from build123d import *

# Parameters (mm, degrees)
PAD002_DEPTH    = 2.5
SKETCH009_W     = 48
SKETCH009_H     = 10.5
PAD003_DEPTH    = 0.4
SKETCH008_R     = 1.4
POCKET005_DEPTH = 5
POCKET012_DEPTH = 5
PAD008_DEPTH    = 0.4


with BuildPart() as part:
    # Sketch007 (on XZ_Plane001 of Origin002) → Pad002 (new body)
    with BuildSketch(Plane.XZ):
        Polygon((50.5, 0), (50.5, 40), (27.253439, 40), (2.5, 10.5), (2.5, 0), align=None)
    extrude(amount=PAD002_DEPTH)

    # Sketch009 (on Face7 of Pad002) → Pad003 (join)
    with BuildSketch(Plane.XZ.offset(2.5)):
        with Locations((26.5, 5.25)):
            Rectangle(SKETCH009_W, SKETCH009_H)
    extrude(amount=PAD003_DEPTH)

    # Sketch008 (on Face6 of Pad002) → Pocket005 (cut)
    with BuildSketch(Plane(origin=(0, 0, 0), x_dir=(-1, 0, 0), z_dir=(0, 1, 0))):
        with Locations((-45, 4)):
            Circle(SKETCH008_R)
        with Locations((-15, 4)):
            Circle(SKETCH008_R)
    extrude(amount=-POCKET005_DEPTH, mode=Mode.SUBTRACT)

    # Sketch021 (on XZ_Plane001 of Origin002) → Pocket012 (cut)
    with BuildSketch(Plane.XZ):
        Polygon((27.253439, 40), (2.5, 10.5), (2.5, 0), (2.8, 0), (2.8, 10.5), (27.553439, 40), align=None)
    extrude(amount=POCKET012_DEPTH, mode=Mode.SUBTRACT)

    # Sketch022 (on Face4 of Pocket012) → Pad008 (join)
    with BuildSketch(Plane.XZ.offset(2.5)):
        Polygon((14.5, 10.5), (50.5, 10.5), (50.5, 14), align=None)
    extrude(amount=PAD008_DEPTH)


solid = part.part
The listing builds one solid part. Answer for the finished solid, in the listing's coordinates (mm). Round coordinates to 2 decimals unless told otherwise and drop trailing zeros. Order: outer loops, then holes, each group sorted by start corner. A loop starts at its lowest first (then second) coordinate and runs counter-clockwise, first axis right, second up. Notation, with made-up numbers: (-19, -31.5) - (5, -31.5) arc R26 cw to (5, 1.5) - close; hole circle Ø8 at (1, 2.5). An arc over 180 degrees is marked (long way). Write item = value, one per line. Start each with the question number.
1) Section A-A, the plane z = 4 is taken. Write down the section's boundary in (x, y).
2) Section C-C, the plane x = 15 is taken. Write down the section's boundary in (y, z).
3) Given pin 1 (3.5 mm diameter, centred on x = 15, z = 4, fed in from +Y); pin 2 (2.5 mm diameter, centred on x = 45, z = 4, fed in from +Y), each flat-ended and moving along its own axis, determine where each tip first touches the part or whether it passes through.
4) Section B-B, the plane y = -1.1 is taken. Write down the section's boundary in (x, z).
5) Section D-D, the plane x = 26.5 is taken. Write down the section's boundary in (y, z), plus the area to 3 significant figures.
6) Straight lines are drawn through the part: L1, parallel to Z at x = 45, y = -0.6; L2, parallel to Y at x = 17, z = 16.5; L3, parallel to Z at x = 15, y = -1.4. For each, find the intervals that lie inside material, in ascending order.
7) For a pull along Z with two mould halves and no side action, classify faces 1 (the cylindrical face through (16.4, -1.43, 4.06)), 2 (the flat face through (26, -1, 0)), 3 (the flat face through (32.752, -2.697, 12.274)), 4 (the cylindrical face through (43.665, -1.43, 4.421)) as released by +Z, released by -Z, zero draft, split by the parting line, or undercut.
Results list:
q1.outline = (2.8, -2.9) - (13.6, -2.9) - (13.6, 0) - (2.8, 0) - close; (16.4, -2.9) - (43.6, -2.9) - (43.6, 0) - (16.4, 0) - close; (46.4, -2.9) - (50.5, -2.9) - (50.5, 0) - (46.4, 0) - close
q2.outline = (-2.9, 0) - (0, 0) - (0, 2.6) - (-2.9, 2.6) - close; (-2.9, 5.4) - (0, 5.4) - (0, 25.04) - (-2.5, 25.04) - (-2.5, 10.55) - (-2.9, 10.55) - close
q3.pin_1 = 0
q3.pin_2 = through
q4.outline = (2.8, 0) - (50.5, 0) - (50.5, 40) - (27.55, 40) - (2.8, 10.5) - close; hole circle Ø2.8 at (15, 4); hole circle Ø2.8 at (45, 4)
q5.outline = (-2.9, 0) - (0, 0) - (0, 38.74) - (-2.5, 38.74) - (-2.5, 11.67) - (-2.9, 11.67) - close
q5.area = 102 mm^2
q6.L1 = 0 to 2.6, 5.4 to 40
q6.L2 = -2.5 to 0
q6.L3 = 0 to 2.6, 5.4 to 25.04
q7.face_1 = undercut
q7.face_2 = released by -Z
q7.face_3 = released by +Z
q7.face_4 = undercut
